For this review, take the finished solid that the model builds, in its own axes (mm). A direction names the side the tool comes from. Give positions to 0.01 mm unless a question says otherwise; leave off trailing zeros. Loops run counter-clockwise (first coordinate to the right, second up) from the corner with the lowest first, then second, coordinate; pieces in that order, holes last. Notation, with made-up numbers: (-9, 7.5) -> (41, 7.5) arc R15 cw to (41, 36.5) -> close; hole circle Ø10 at (79.25, -34.5). An arc over 180 degrees is marked (long way). Answer as CSV lines item,"result". Start each with the question number.
Item 1: Machinability: for faces 1 (the face through (51, -35.5, -7)), 2 (the face through (51, -34.5, -7)), 3 (the face through (49, -40.5, 99)), which of the approach directions +Z, -Z, +X, -X, +Y, -Y give a long, thin tool a straight path to every point of the face, cutting with its end or side? Answer none if there is none.
Item 2: Clearance check with flat-ended pins moving along their axes: P1, Ø4, axis at x = 87, y = -33, coming from the -Z side; P2, Ø0.9, axis at y = -23.5, z = 202, coming from the +X side; P3, Ø12, axis at x = 41, y = -35, coming from the +Z side; P4, Ø2, axis at x = 5, y = -20.3, coming from the -Z side. State where each tip first meets the part, or that it passes through.
Item 3: The part is to be moulded in two halves that separate along X. For faces 4 (the face through (100, -21, 91)), 5 (the face through (0, -21, 91)), 6 (the face through (65, -22, 200)), 7 (the face through (49, 0, 99)), say which applies: +X half, -X half, draft (parallel to the pull), parting line (faces both ways), or undercut.
Item 4: Add section B-B on x = 20. State the section outline as (y, z) points.
Item 5: Add section A-A on y = -25. State the section outline as (x, z) points.
Item 6: For L1, parallel to X at y = -20, z = 197; L2, parallel to Z at x = 15, y = -35; L3, parallel to Z at x = 96, y = -3, list the stretches that pass through material, from the lowest coordinate up. Write a range as from..to.
```python
from build123d import *

# Parameters (mm, degrees)
SKETCH1_W          = 100
SKETCH1_H          = 40.5
EXTRUDE1_DEPTH     = 200
SKETCH2_R          = 1.778
CUT_EXTRUDE1_DEPTH = 10
SKETCH3_W          = 100
SKETCH3_H          = 1
EXTRUDE2_DEPTH     = 15
SKETCH4_R          = 1.778
CUT_EXTRUDE2_DEPTH = 15
SKETCH5_W          = 11.629297252
SKETCH5_H          = 23.097430101
EXTRUDE3_DEPTH     = 3
SKETCH6_W          = 7.618566084
SKETCH6_H          = 17.291576956
CUT_EXTRUDE3_DEPTH = 3


with BuildPart() as part:
    # Sketch1 → Extrude1 (new body)
    with BuildSketch(Plane.XY):
        with Locations((50, -20.25)):
            Rectangle(SKETCH1_W, SKETCH1_H)
    extrude(amount=EXTRUDE1_DEPTH)

    # Sketch2 → Cut-Extrude1 (cut)
    with BuildSketch(Plane.XY.offset(200)):
        with Locations((95, -20.3)):
            Circle(SKETCH2_R)
        with Locations((5, -20.3)):
            Circle(SKETCH2_R)
    extrude(amount=-CUT_EXTRUDE1_DEPTH, mode=Mode.SUBTRACT)

    # Sketch3 → Extrude2 (add)
    with BuildSketch(Plane(origin=(0, 0, 0), x_dir=(-1, 0, 0), z_dir=(0, 0, -1))):
        with Locations((-50, -35)):
            Rectangle(SKETCH3_W, SKETCH3_H)
    extrude(amount=EXTRUDE2_DEPTH)

    # Sketch4 → Cut-Extrude2 (cut)
    with BuildSketch(Plane(origin=(0, -34.5, 0), x_dir=(-1, 0, 0), z_dir=(0, 1, 0))):
        with Locations((-15, -11)):
            Circle(SKETCH4_R)
        with Locations((-85, -11)):
            Circle(SKETCH4_R)
    extrude(amount=-CUT_EXTRUDE2_DEPTH, mode=Mode.SUBTRACT)

    # Sketch5 → Extrude3 (add)
    with BuildSketch(Plane.XY.offset(200)):
        with Locations((65.188803726, -22.404247031)):
            Rectangle(SKETCH5_W, SKETCH5_H)
    extrude(amount=EXTRUDE3_DEPTH)

    # Sketch6 → Cut-Extrude3 (cut)
    with BuildSketch(Plane.XY.offset(203)):
        with Locations((65.10872937, -22.176041988)):
            Rectangle(SKETCH6_W, SKETCH6_H)
    extrude(amount=-CUT_EXTRUDE3_DEPTH, mode=Mode.SUBTRACT)


solid = part.part
```
Computed values:
1,face 1,"-Z, +X, -X, -Y"
1,face 2,"-Z, +X, -X, +Y"
1,face 3,"+Z, -Z, +X, -X, -Y"
2,P1,"z = -15"
2,P2,"x = 71"
2,P3,"z = 200"
2,P4,"z = 0"
3,face 4,"+X half"
3,face 5,"-X half"
3,face 6,"undercut"
3,face 7,"draft"
4,outline,"(-40.5, 0) -> (-35.5, 0) -> (-35.5, -15) -> (-34.5, -15) -> (-34.5, 0) -> (0, 0) -> (0, 200) -> (-40.5, 200) -> close"
5,outline,"(0, 0) -> (100, 0) -> (100, 200) -> (71, 200) -> (71, 203) -> (68.92, 203) -> (68.92, 200) -> (61.3, 200) -> (61.3, 203) -> (59.37, 203) -> (59.37, 200) -> (0, 200) -> close"
6,L1,"0..3.25, 6.75..93.25, 96.75..100"
6,L2,"-15..-12.78, -9.22..200"
6,L3,"0..200"
